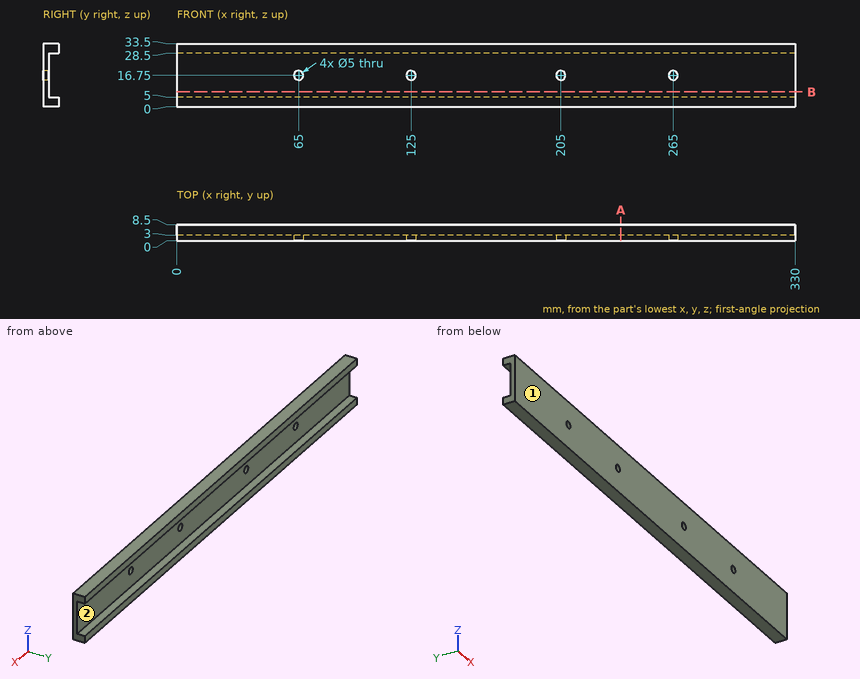
Print and shaded views of the part. All mm, measured from the part's lowest x, y and z. Give positions to 0.01 mm unless a question says otherwise; leave off trailing zeros. Write each loop counter-clockwise with the first axis right and the second up, starting at its lowest first coordinate (ties: lowest second). Pieces come first, ordered by that corner, then holes. Notation, with made-up numbers: (27, 32) -> (46, 32) arc R21 cw to (46, 61) -> close; hole circle Ø2 at (39.25, -22). An arc over 180 degrees is marked (long way). Use CSV: the item, a comma, the result in double quotes. Start each with the question number.
1) Cut at A-A on x = 237. List the corners of the cut face in (y, z).
2) Two-plate mould, pull along Z, no slides. Class the marked faces 1 and 2: released by +Z, released by -Z, zero draft, split by the parting line, or undercut.
3) Cut at B-B on z = 8. List the corners of the cut face in (x, y).
4) Drill centre lines: L1, parallel to X at y = 1.45, z = 16.75; L2, parallel to Z at x = 115, y = 4.5; L3, parallel to Z at x = 125, y = 1.1. Where is each one in solid material? Low to high.
5) Pin check, flat tips, straight feed: P1, Ø1, axis at y = 5, z = 17, coming from the +X side; P2, Ø6.5, axis at x = 205, z = 16.75, coming from the +Y side. Stop position of each tip, or through.
Final values:
1,outline,"(0, 0) -> (8.5, 0) -> (8.5, 5) -> (3, 5) -> (3, 28.5) -> (8.5, 28.5) -> (8.5, 33.5) -> (0, 33.5) -> close"
2,face 1,"zero draft"
2,face 2,"undercut"
3,outline,"(0, 0) -> (330, 0) -> (330, 3) -> (0, 3) -> close"
4,L1,"x = 0 to 62.5, 67.5 to 122.5, 127.5 to 202.5, 207.5 to 262.5, 267.5 to 330"
4,L2,"z = 0 to 5, 28.5 to 33.5"
4,L3,"z = 0 to 14.25, 19.25 to 33.5"
5,P1,"passes through"
5,P2,"stops at y = 3"
